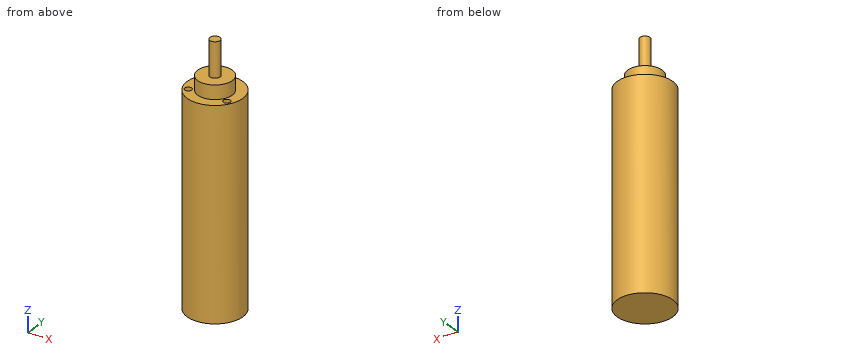
from build123d import *

# Parameters (mm, degrees)
SKETCH1_R           = 8.05
BOSS_EXTRUDE1_DEPTH = 60
SKETCH2_R           = 5
BOSS_EXTRUDE2_DEPTH = 4
SKETCH3_R           = 1
CUT_EXTRUDE1_DEPTH  = 5
SKETCH4_R           = 1.5
BOSS_EXTRUDE3_DEPTH = 10


with BuildPart() as part:
    # Sketch1 → Boss-Extrude1 (new body)
    with BuildSketch(Plane.XY):
        Circle(SKETCH1_R)
    extrude(amount=BOSS_EXTRUDE1_DEPTH)

    # Sketch2 → Boss-Extrude2 (add)
    with BuildSketch(Plane.XY.offset(60)):
        Circle(SKETCH2_R)
    extrude(amount=BOSS_EXTRUDE2_DEPTH)

    # Sketch3 → Cut-Extrude1 (cut)
    with BuildSketch(Plane.XY.offset(60)):
        with Locations((0, 6.5)):
            Circle(SKETCH3_R)
        with Locations((5.629165125, -3.25)):
            Circle(SKETCH3_R)
        with Locations((-5.629165125, -3.25)):
            Circle(SKETCH3_R)
    extrude(amount=-CUT_EXTRUDE1_DEPTH, mode=Mode.SUBTRACT)

    # Sketch4 → Boss-Extrude3 (add)
    with BuildSketch(Plane.XY.offset(64)):
        Circle(SKETCH4_R)
    extrude(amount=BOSS_EXTRUDE3_DEPTH)


solid = part.part
Check sheet for the modelled part. Datum: model origin and axes. Units: mm. Round coordinates to 2 decimals unless told otherwise and drop trailing zeros. Write each loop counter-clockwise with the first axis right and the second up, starting at its lowest first coordinate (ties: lowest second). Pieces come first, ordered by that corner, then holes. Notation, with made-up numbers: (-25.75, 19.25) -> (22.25, 19.25) arc R10 cw to (22.25, 28.25) -> close; hole circle Ø1 at (85, 7.5). An arc over 180 degrees is marked (long way). Answer as CSV lines item,"result". Start each with the question number.
1) Section check D-D on x = 3.75. Enter the section's corners in (y, z).
2) Material ranges on line 1 (Z direction, x = -2.75, y = 1); line 2 (Z direction, x = -0.25, y = 6.25); line 3 (Y direction, x = 4.25, z = 44), recorded low to high. Write a range as from..to.
3) Section check C-C on z = 56.5. Enter the section's corners in (x, y), and give its area (3 significant figures).
4) Section check A-A on y = 0. Enter the section's corners in (x, z), and give its area (3 significant figures).
5) Go/stop test with flat-tipped pins: P1, Ø1, axis at x = -5.5, y = -3.5, coming from the +Z side; P2, Ø1.6, axis at x = 5, y = -3, coming from the +Z side; P3, Ø4, axis at y = -4, z = 56.5, coming from the -X side. Record where each tip stops, or that it passes through.
6) Section check B-B on x = 0. Enter the section's corners in (y, z), and give its area (3 significant figures).
Found:
1,outline,"(-7.12, 0) -> (7.12, 0) -> (7.12, 60) -> (3.31, 60) -> (3.31, 64) -> (-3.31, 64) -> (-3.31, 60) -> (-7.12, 60) -> close"
2,line 1,"z = 0..64"
2,line 2,"z = 0..55"
2,line 3,"y = -6.84..6.84"
3,outline,"circle Ø16.1 at (0, 0); hole circle Ø2 at (-5.63, -3.25); hole circle Ø2 at (0, 6.5); hole circle Ø2 at (5.63, -3.25)"
3,area,"194 mm^2"
4,outline,"(-8.05, 0) -> (8.05, 0) -> (8.05, 60) -> (5, 60) -> (5, 64) -> (1.5, 64) -> (1.5, 74) -> (-1.5, 74) -> (-1.5, 64) -> (-5, 64) -> (-5, 60) -> (-8.05, 60) -> close"
4,area,"1,040 mm^2"
5,P1,"stops at z = 55"
5,P2,"stops at z = 60"
5,P3,"stops at x = -7.8"
6,outline,"(-8.05, 0) -> (8.05, 0) -> (8.05, 60) -> (7.5, 60) -> (7.5, 55) -> (5.5, 55) -> (5.5, 60) -> (5, 60) -> (5, 64) -> (1.5, 64) -> (1.5, 74) -> (-1.5, 74) -> (-1.5, 64) -> (-5, 64) -> (-5, 60) -> (-8.05, 60) -> close"
6,area,"1,030 mm^2"
